Work out the finished part from the listing and answer in its coordinate system (mm). Face numbers are marked on the shaded views. A direction names the side the tool comes from. Give positions to 0.01 mm unless a question says otherwise; leave off trailing zeros. Loops run counter-clockwise (first coordinate to the right, second up) from the corner with the lowest first, then second, coordinate; pieces in that order, holes last. Notation, with made-up numbers: (31.5, -2) - (84.5, -2) arc R18 cw to (84.5, 3) - close; hole circle Ø4 at (28, -40). An arc over 180 degrees is marked (long way). One line per item, written item: value.
Autodesk Inventor part; units mm, degrees
ref_plane "Work Plane1" through (173.3333, 20, -7) normal (1, 0, 0) x (0, 0, -1)
ref_plane "Work Plane2" through (86.6667, 20, -7) normal (1, 0, 0) x (0, 0, -1)
ref_plane "YZ Plane" through (0, 0, 0) normal (1, 0, 0) x (0, 1, 0)
sketch "Sketch1" plane through (0, 0, 0) normal (0, 0, 1) x (1, 0, 0)
  line L0 (0, 0) -> (260, 0)
  line L1 (260, 0) -> (260, 20)
  line L2 (260, 20) -> (0, 20)
  line L3 (0, 20) -> (0, 0)
  dimension "d0" = 260
  dimension "d1" = 20
extrude "Extrusion1" add sketch "Sketch1" along normal blind 3
sketch "Sketch2" plane through (0, 0, 0) normal (0, 0, -1) x (-1, 0, 0)
  line L0 (0, 0) -> (-260, 0)
  line L1 (-12.5251, -24.7625) -> (-37.9251, -24.7625)
  line L2 (-260, 20) -> (0, 20)
  point P0 (-25.2251, 30)
  dimension "d5" = 25.4
  dimension "d6" = 12.7
  dimension "d62" = 10
sketch "Sketch5" plane through (0, 0, 0) normal (-1, 0, 0) x (0, 0, 1)
  line L0 (0, 20) -> (3, 20)
  line L1 (3, 20) -> (-7, 20)
  line L2 (-7, 20) -> (-7, 40)
  line L3 (-7, 40) -> (3, 40)
  line L4 (3, 40) -> (3, 20)
  point P0 (0, 0)
  point P1 (3, 30)
  point P2 (1.5, 20)
  dimension "d31" = 10
  dimension "d32" = 20
extrude "Extrusion3" add sketch "Sketch5" against normal up to surface (260 mm away)
sketch "Sketch6" plane through (0, 0, 3) normal (0, 0, 1) x (1, 0, 0)
  line L0 (0, 0) -> (0, 40)
  line L1 (260, 0) -> (260, 40)
  line L2 (0, 40) -> (260, 40)
  point P0 (42.6875, 30)
  point P1 (77.6125, 30)
  point P2 (182.3875, 30)
  point P3 (217.3125, 30)
  point P4 (112.5375, 30)
  point P5 (147.4625, 30)
  dimension "d35" = 42.6875
  dimension "d46" = 42.6875
  dimension "d47" = 34.925
  dimension "d48" = 34.925
  dimension "d49" = 34.925
  dimension "d50" = 34.925
  dimension "d51" = 10
hole "Hole2" at (42.6875, 30, 3) at (77.6125, 30, 3) at (182.3875, 30, 3) at (217.3125, 30, 3) at (112.5375, 30, 3) at (147.4625, 30, 3) direction (0, 0, -1) diameter 6 end through all
hole "Hole3" at (25.2251, 30, 0) direction (0, 0, 1) diameter 4.3 depth 6
pattern_linear "Rectangular Pattern2" count 7 spacing 34.925 along (1, 0, 0) of "Hole3"
chamfer "Chamfer1" distance 2 angle 45 1 edges at (130, 20, 0)
sketch "Sketch7" plane through (0, 0, 0) normal (-1, 0, 0) x (0, 0, 1)
  line L0 (0, 0) -> (3, 0)
  line L1 (0, 0) -> (3.6796, 0)
  line L2 (3.6796, 0) -> (3.6796, 5)
  line L3 (3.6796, 5) -> (0, 5)
  line L4 (0, 5) -> (0, 0)
  dimension "d66" = 5
extrude "Extrusion4" cut sketch "Sketch7" against normal through all
ref_plane "Work Plane1" through (173.3333, 20, -7) normal (1, 0, 0) x (0, 0, -1)
ref_plane "Work Plane2" through (86.6667, 20, -7) normal (1, 0, 0) x (0, 0, -1)
sketch "Sketch8" plane through (173.3333, 20, -7) normal (1, 0, 0) x (0, 0, -1)
  line L0 (-10, -15) -> (-7, -15)
  line L1 (-7, -15) -> (-7, -2)
  line L2 (-5, 0) -> (-7, -2)
  line L3 (0, 0) -> (-5, 0)
  line L4 (0, 20) -> (0, 0)
  line L5 (-10, 20) -> (0, 20)
  line L6 (-10, -15) -> (-10, 20)
  point P0 (-7, -20)
extrude "Extrusion5" cut sketch "Sketch8" along normal through all
sketch "Sketch9" plane through (86.6667, 20, -7) normal (1, 0, 0) x (0, 0, -1)
  line L0 (0, 13) -> (-10, 13)
  line L1 (-7, -15) -> (-10, -15)
  line L2 (-7, -2) -> (-7, -15)
  line L3 (-5, 0) -> (-7, -2)
  line L4 (0, 0) -> (-5, 0)
  line L5 (0, 20) -> (0, 0)
  line L6 (-10, 20) -> (0, 20)
  line L7 (-10, -15) -> (-10, 20)
  point P0 (-7, -20)
extrude "Extrusion6" cut sketch "Sketch9" against normal through all
properties part number "IR_Mount_Plate_3DPrint"
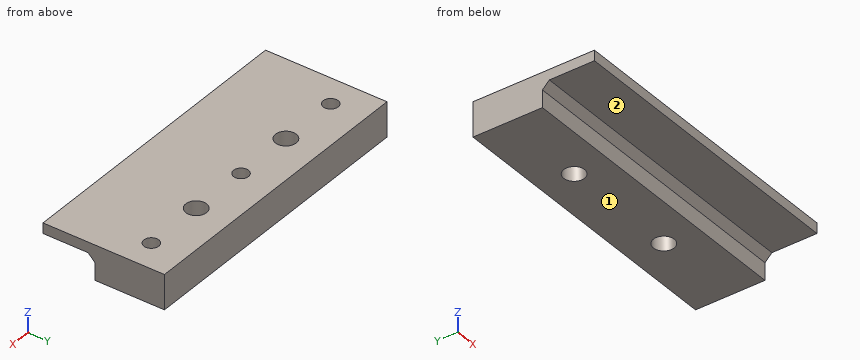
1. Section D-D (z = -1) is taken. Write down the section's boundary in (x, y).
Output:
outline: (86.67, 19) - (173.33, 19) - (173.33, 40) - (86.67, 40) - close; hole circle Ø6 at (112.54, 30); hole circle Ø6 at (147.46, 30)
2. Flat-ended cylindrical pins translate along their axes: pin 1 Ø12 at (x, y) = (122, 10.5) entering from -Z; pin 2 Ø1.3 at (x, y) = (94, 30.5) entering from +Z; pin 3 Ø6 at (y, z) = (11.5, -3.5) entering from +X; pin 4 Ø1.5 at (x, z) = (129.5, -5.5) entering from -Y. Find the tip coordinate at first contact, or state that the pin passes through.
Output:
pin 1: stops at z = 0
pin 2: stops at z = 0
pin 3: passes through
pin 4: stops at y = 20
3. For the marked faces 1 and 2, determine the directions among +Z, -Z, +X, -X, +Y, -Y from which every point of the face is accessible in a straight line to the end or side of a thin tool.
Output:
face 1: -Z, +X, -X, +Y, -Y
face 2: -Z, +X, -X, -Y
4. Section B-B (x = 113.5) is taken. Write down the section's boundary in (y, z).
Output:
outline: (5, 0) - (18, 0) - (20, -2) - (20, -7) - (27.16, -7) - (27.16, 3) - (5, 3) - close; (32.84, -7) - (40, -7) - (40, 3) - (32.84, 3) - close
5. Section C-C (x = 101.5) is taken. Write down the section's boundary in (y, z).
Output:
outline: (5, 0) - (18, 0) - (20, -2) - (20, -7) - (40, -7) - (40, 3) - (5, 3) - close
6. Section A-A (y = 30) is taken. Write down the section's boundary in (x, z), and give its area (3 significant figures).
Output:
outline: (86.67, -7) - (109.54, -7) - (109.54, 3) - (97.23, 3) - (97.23, 0) - (92.93, 0) - (92.93, 3) - (86.67, 3) - close; (115.54, -7) - (144.46, -7) - (144.46, 3) - (132.15, 3) - (132.15, 0) - (127.85, 0) - (127.85, 3) - (115.54, 3) - close; (150.46, -7) - (173.33, -7) - (173.33, 3) - (167.08, 3) - (167.08, 0) - (162.78, 0) - (162.78, 3) - (150.46, 3) - close
area: 708 mm²
7. Find the intervals of material crossed by line 1 along X through (y, z) = (30, -4.25); line 2 along X through (y, z) = (30, 0.75); line 3 along X through (y, z) = (28.5, -1.25), in increasing order.
Output:
line 1: x = 86.67 to 109.54, 115.54 to 144.46, 150.46 to 173.33
line 2: x = 86.67 to 92.93, 97.23 to 109.54, 115.54 to 127.85, 132.15 to 144.46, 150.46 to 162.78, 167.08 to 173.33
line 3: x = 86.67 to 109.94, 115.14 to 144.86, 150.06 to 173.33
